Read the model definition and answer for the solid it produces. Units are mm, in the model's axes. A direction names the side the tool comes from. Coordinates: 2 decimals unless noted, no trailing zeros. Write each loop counter-clockwise with the first axis right and the second up, starting at its lowest first coordinate (ties: lowest second). Pieces come first, ordered by that corner, then holes.
Item 1: A tool of negligible diameter and unlimited length cuts with its end or side. For faces 4 (the face through (-30, -0.8, 3.53)), 5 (the face through (-33.563, -6.157, -32.435)), 6 (the face through (30, -0.8, -34.97)), 7 (the face through (29.095, 2.414, -52.217)), from which of +Z, -Z, +X, -X, +Y, -Y can it reach the whole face along a straight path? Write none if from no direction.
Item 2: Determine the mould class of faces 1 (the face through (-24.9, -1, 6)), 2 (the face through (-30, -0.8, -29.97)), 3 (the face through (35, -2, 6)) for opening direction X: released by +X, released by -X, zero draft, split by the parting line, or undercut.
Item 3: Section B-B (x = -15) is taken. Give the vertices of the cut face in (y, z), then the cut area to 3 significant figures.
Item 4: Section C-C (y = 0.25) is taken. Give the vertices of the cut face in (x, z), then the cut area to 3 significant figures.
Item 5: Straight lines are drawn through the part: probe 1 along X at (y, z) = (-4.1, -32.65); probe 2 along Z at (x, y) = (-35.5, 3); probe 3 along Z at (x, y) = (-30.5, 0.75). For each, find the intervals that lie inside material, in ascending order.
Item 6: Each of these flat-tipped pins is pushed along its axis until it touches: P1, Ø2.5, axis at x = 32, y = -4.5, coming from the +Z side; P2, Ø1, axis at x = 28.5, z = 4.5, coming from the +Y side; P3, Ø2.5, axis at y = -2, z = 6, coming from the +X side. Where does it stop, or does it pass through?
Item 7: Section A-A (z = -46.5) is taken. Give the vertices of the cut face in (x, y).
Item 8: Section D-D (x = -28.5) is taken. Give the vertices of the cut face in (y, z).
from build123d import *

# Parameters (mm, degrees)
SKETCH1_W               = 70
SKETCH1_H               = 57.5
BOSS_EXTRUDE1_DEPTH     = 8
BOSS_EXTRUDE2_START     = -2
SKETCH3_R               = 3.1
BOSS_EXTRUDE2_DEPTH     = 5
CUT_EXTRUDE1_DEPTH      = 10
CUT_EXTRUDE1_DEPTH_BACK = 63
MOVE_FACE1_BY           = 6
SKETCH5_W               = 80
SKETCH5_H               = 80
BOSS_EXTRUDE3_DEPTH     = 2
FILLET1_R               = 2
SKETCH6_R               = 2.275
CUT_EXTRUDE2_DEPTH      = 2
SKETCH7_W               = 60.186291501
SKETCH7_H               = 60.186291501
CUT_EXTRUDE3_DEPTH      = 2
FILLET2_R               = 4


with BuildPart() as part:
    # Sketch1 → Boss-Extrude1 (new body)
    with BuildSketch(Plane(origin=(0, 1.4, 0), x_dir=(1, 0, 0), z_dir=(0, 1, 0))):
        with Locations((0, 12.22)):
            Rectangle(SKETCH1_W, SKETCH1_H)
    extrude(amount=BOSS_EXTRUDE1_DEPTH)

    # Sketch3 → Boss-Extrude2 (add)
    # profile 1 of 2: a face of its own
    with BuildSketch(Plane(origin=(0, 0, -36.97), x_dir=(-1, 0, 0), z_dir=(0, 0, -1)).offset(BOSS_EXTRUDE2_START)):
        with BuildLine():
            ThreePointArc((-35, -5.104987562), (-29.495024753, -9.174938423), (-24.9, -4.1))
            Line((-24.9, -4.1), (-24.9, 1.4))
            Line((-24.9, 1.4), (-35, 1.4))
            Line((-35, 1.4), (-35, -5.104987562))
        make_face()
        with Locations(Location((-30, -4.1, 0), (0, 0, 180))):
            Circle(SKETCH3_R, mode=Mode.SUBTRACT)
    # profile 2 of 2: a face of its own
    with BuildSketch(Plane(origin=(0, 0, -36.97), x_dir=(-1, 0, 0), z_dir=(0, 0, -1)).offset(BOSS_EXTRUDE2_START)):
        with BuildLine():
            Line((35, 1.4), (35, -5.104987562))
            ThreePointArc((35, -5.104987562), (29.495024753, -9.174938423), (24.9, -4.1))
            Line((24.9, -4.1), (24.9, 1.4))
            Line((24.9, 1.4), (35, 1.4))
        make_face()
        with Locations(Location((30, -4.1, 0), (0, 0, 180))):
            Circle(SKETCH3_R, mode=Mode.SUBTRACT)
    boss_extrude2 = extrude(amount=-BOSS_EXTRUDE2_DEPTH)

    # Mirror1: Boss-Extrude2 across plane
    add(boss_extrude2.mirror(Plane.XY.offset(-13.22)))

    # Sketch4 → Cut-Extrude1 (cut, two sides: drawn at the far end of the back side and taken through both)
    with BuildSketch(Plane(origin=(0, 0, -29.97), x_dir=(-1, 0, 0), z_dir=(0, 0, -1)).offset(-CUT_EXTRUDE1_DEPTH_BACK)):
        Polygon((-30, -4.1), (-20, -9.873502692), (-40, -9.873502692), align=None)
        Polygon((20, -9.873502692), (40, -9.873502692), (30, -4.1), align=None)
    extrude(amount=CUT_EXTRUDE1_DEPTH + CUT_EXTRUDE1_DEPTH_BACK, mode=Mode.SUBTRACT)

    # Move Face1: a face moved inward by 6.0
    extrude(part.faces().sort_by_distance((0, 9.4, -12.22))[0], amount=MOVE_FACE1_BY, dir=(0, -1, 0), mode=Mode.SUBTRACT)

    # Sketch5 → Boss-Extrude3 (add)
    with BuildSketch(Plane(origin=(0, 3.4, 0), x_dir=(1, 0, 0), z_dir=(0, 1, 0))):
        with Locations((0, 23.47)):
            Rectangle(SKETCH5_W, SKETCH5_H)
    extrude(amount=-BOSS_EXTRUDE3_DEPTH)

    # Fillet1
    fillet1_edges = [part.edges().sort_by_distance(p)[0] for p in [
        (40, 2.4, 16.53),
        (-40, 2.4, 16.53),
        (-40, 2.4, -63.47),
        (40, 2.4, -63.47),
    ]]
    fillet(fillet1_edges, radius=FILLET1_R)

    # Sketch6 → Cut-Extrude2 (cut)
    with BuildSketch(Plane(origin=(0, 3.4, 0), x_dir=(1, 0, 0), z_dir=(0, 1, 0))):
        with Locations(Location((35.955095469, 59.014904531, 0), (0, 0, 180))):
            Circle(SKETCH6_R)
        with Locations(Location((35.955095469, -12.485095469, 0), (0, 0, 180))):
            Circle(SKETCH6_R)
        with Locations(Location((-35.544904531, 59.014904531, 0), (0, 0, 180))):
            Circle(SKETCH6_R)
        with Locations(Location((-35.544904531, -12.485095469, 0), (0, 0, 180))):
            Circle(SKETCH6_R)
    extrude(amount=-CUT_EXTRUDE2_DEPTH, mode=Mode.SUBTRACT)

    # Sketch7 → Cut-Extrude3 (cut)
    with BuildSketch(Plane(origin=(0, 3.4, 0), x_dir=(1, 0, 0), z_dir=(0, 1, 0))):
        with Locations((0.205095468, 23.264904532)):
            Rectangle(SKETCH7_W, SKETCH7_H)
    extrude(amount=-CUT_EXTRUDE3_DEPTH, mode=Mode.SUBTRACT)

    # Fillet2
    # the kernel refuses this fillet: 4 mm, written as the material it adds along each edge
    with BuildSketch(Plane(origin=(30.298241219, 3.4, -53.358050282), x_dir=(-1, 0, 0), z_dir=(0, -1, 0)), Plane(origin=(30.298241219, 3.4, 6.828241219), x_dir=(0, 0, -1), z_dir=(0, -1, 0)), Plane(origin=(-29.888050282, 3.4, -53.358050282), x_dir=(0, 0, 1), z_dir=(0, -1, 0))) as fillet2_piece_1:
        with BuildLine():
            CenterArc((FILLET2_R, -FILLET2_R), FILLET2_R, 90, 90)
            Line((0, -FILLET2_R), (0, 0))
            Line((0, 0), (FILLET2_R, 0))
        make_face()
    extrude(amount=2)
    with BuildSketch(Plane(origin=(-29.888050282, 3.4, 6.828241219), x_dir=(0, 0, -1), z_dir=(0, -1, 0))) as fillet2_piece_2:
        with BuildLine():
            CenterArc((FILLET2_R, FILLET2_R), FILLET2_R, 180, 90)
            Line((0, FILLET2_R), (0, 0))
            Line((0, 0), (FILLET2_R, 0))
        make_face()
    extrude(amount=2)


solid = part.part
Established:
1. face 4: +X, -X, -Y
1. face 5: +Z, -Z, -Y
1. face 6: -Z, +X, -X, -Y
1. face 7: +Y, -Y
2. face 1: undercut
2. face 2: zero draft
2. face 3: released by +X
3. outline: (1.4, -63.47) - (3.4, -63.47) - (3.4, -53.36) - (1.4, -53.36) - close; (1.4, 6.83) - (3.4, 6.83) - (3.4, 16.53) - (1.4, 16.53) - close
3. area: 39.6 mm2
4. outline: (-35, -34.97) - (-24.9, -34.97) - (-24.9, -29.97) - (-35, -29.97) - close; (-35, 3.53) - (-24.9, 3.53) - (-24.9, 8.53) - (-35, 8.53) - close; (24.9, -34.97) - (35, -34.97) - (35, -29.97) - (24.9, -29.97) - close; (24.9, 3.53) - (35, 3.53) - (35, 8.53) - (24.9, 8.53) - close
4. area: 202 mm2
5. probe 1: x = -35 to -33.1, -26.9 to -24.9, 24.9 to 26.9, 33.1 to 35
5. probe 2: z = -63.47 to -61.29, -56.74 to 10.21, 14.76 to 16.53
5. probe 3: z = -34.97 to -29.97, 3.53 to 8.53
6. P1: stops at z = 8.53
6. P2: stops at y = 1.4
6. P3: stops at x = 35
7. outline: (-40, 1.4) - (-29.89, 1.4) - (-29.89, 3.4) - (-40, 3.4) - close; (30.3, 1.4) - (40, 1.4) - (40, 3.4) - (30.3, 3.4) - close
8. outline: (-1.39, -34.97) - (1.4, -34.97) - (1.4, -29.97) - (-1.39, -29.97) - close; (-1.39, 3.53) - (1.4, 3.53) - (1.4, 5.86) - (3.4, 5.86) - (3.4, 16.53) - (1.4, 16.53) - (1.4, 8.53) - (-1.39, 8.53) - close; (1.4, -63.47) - (3.4, -63.47) - (3.4, -52.39) - (1.4, -52.39) - close
